Read the model definition and answer for the solid it produces. Units are mm, in the model's axes. Coordinates: 2 decimals unless noted, no trailing zeros. Write each loop counter-clockwise with the first axis right and the second up, starting at its lowest first coordinate (ties: lowest second). Pieces come first, ordered by that corner, then holes. Notation, with made-up numbers: (85.25, 34) -> (104.25, 34) arc R27 ccw to (104.25, 55) -> close; hole circle Ø3 at (-18, -30). An arc over 180 degrees is marked (long way). One line per item, written item: value. Start each with the question number.
1. Consider line 1 along Z through (x, y) = (0, -61.5) (3 decimals); line 2 along Y through (x, z) = (7, -19) (3 decimals); line 3 along X through (y, z) = (-21.5, -21.5). Determine where each line is inside the solid, lowest interval first.
2. Given P1, Ø21, axis at x = -14, z = -13, coming from the -Y side (3 decimals); P2, Ø6, axis at y = -25.5, z = -5, coming from the +X side; P3, Ø5, axis at y = -98, z = -13.5, coming from the -X side, each flat-ended and moving along its own axis, determine where each tip first touches the part or whether it passes through.
3. Find section B-B, the plane z = 0. Write down the section's boundary in (x, y) (3 decimals), and give its area (3 significant figures).
4. For a pull along Z with two mould halves and no side action, classify faces 1 (the cylindrical face through (-30.235, -58.724, -23.183)), 2 (the flat face through (0, -9.525, 0)), 3 (the flat face through (-1, 0, 1)) as pulls with the +Z half, pulls with the -Z half, needs draft (parallel to the pull), parting line crosses it, or undercut.
5. Find section A-A, the plane x = 0. Write down the section's boundary in (y, z) (3 decimals), and give its area (3 significant figures).
6. Find section C-C, the plane y = -48. Write down the section's boundary in (x, z) (3 decimals).
```python
from build123d import *

# Parameters (mm, degrees)
F0_R     = 38.1
F0_R_2   = 34.925
F1_DEPTH = 123.825
F2_R     = 34.925
F3_DEPTH = 9.525


# Not quite as in the source:
# - a fillet or chamfer that OpenCascade refuses, or shapes differently, is made with other operations: its cross-section is extruded or revolved along the edge and cut away or added


with BuildPart() as f1:
    # F0 (on Front) → F1 (new body)
    with BuildSketch(Plane.XZ):
        Circle(F0_R)
        Circle(F0_R_2, mode=Mode.SUBTRACT)
    extrude(amount=F1_DEPTH)

    # F2 (on Front) → F3 (join)
    with BuildSketch(Plane.XZ):
        Circle(F2_R)
    extrude(amount=F3_DEPTH)

    # F4: fillet of radius 5.08 on 1 edges, made by hand

    # F4_s1 → F4_t2 (revolve, cut)
    with BuildSketch(Plane.XY):
        with BuildLine():
            ThreePointArc((38.1, -119.1157139607), (37.2321134838, -121.9555202921), (34.925, -123.825))
            Line((34.925, -123.825), (38.1, -123.825))
            Line((38.1, -123.825), (38.1, -119.1157139607))
        make_face()
    revolve(axis=Axis((0, -123.825, 0), (0, -1, 0)), mode=Mode.SUBTRACT)


solid = f1.part
```
Answer block:
1. line 1: z = -38.1 to -34.925, 34.925 to 38.1
1. line 2: y = -9.525 to 0
1. line 3: x = -31.45 to -27.52, 27.52 to 31.45
2. P1: stops at y = -9.525
2. P2: stops at x = 38.05
2. P3: stops at x = -36.48
3. outline: (-38.1, -119.116) arc R5.08 ccw to (-34.925, -123.825) -> (-34.925, -9.525) -> (34.925, -9.525) -> (34.925, -123.825) arc R5.08 ccw to (38.1, -119.116) -> (38.1, 0) -> (-38.1, 0) -> close
3. area: 1,440 mm2
4. face 1: parting line crosses it
4. face 2: undercut
4. face 3: needs draft
5. outline: (-123.825, -34.925) arc R5.08 ccw to (-119.116, -38.1) -> (0, -38.1) -> (0, 38.1) -> (-119.116, 38.1) arc R5.08 ccw to (-123.825, 34.925) -> (-9.525, 34.925) -> (-9.525, -34.925) -> close
5. area: 1,440 mm2
6. outline: circle Ø76.2 at (0, 0); hole circle Ø69.85 at (0, 0)
